For this review, take the finished solid that the model builds, in its own axes (mm). Give positions to 0.01 mm unless a question says otherwise; leave off trailing zeros. Write each loop counter-clockwise with the first axis right and the second up, starting at its lowest first coordinate (ties: lowest second). Pieces come first, ordered by that corner, then holes. Notation, with made-up numbers: (0, 28) -> (35, 28) arc R13 ccw to (35, 42) -> close; hole circle Ø2 at (-21.5, 23). An arc over 180 degrees is marked (long way). Answer as CSV lines item,"result".
Autodesk Inventor part; units mm, degrees
ref_plane "YZ Plane" through (0, 0, 0) normal (1, 0, 0) x (0, 1, 0)
ref_plane "XZ Plane" through (0, 0, 0) normal (0, 1, 0) x (-1, 0, 0)
ref_plane "XY Plane" through (0, 0, 0) normal (0, 0, 1) x (1, 0, 0)
sketch "Sketch1" plane through (0, 0, 0) normal (0, 1, 0) x (-1, 0, 0)
  line L0 (0, 0) -> (1000, 0)
  line L1 (1000, 0) -> (1000, 1500)
  line L2 (1000, 1500) -> (0, 1500)
  line L3 (0, 1500) -> (0, 0)
  dimension "d0" = 1000
  dimension "d1" = 1500
extrude "base" add sketch "Sketch1" along normal blind 150
sketch "Sketch2" plane through (0, 150, 0) normal (0, 1, 0) x (1, 0, 0)
  circle A0 centre (-290, -609) radius 55
  line L0 (0, 0) -> (-1000, 0)
  line L1 (0, -1500) -> (0, 0)
  dimension "d4" = 110
  dimension "d38" = 609
  dimension "d62" = 290
extrude "air" cut sketch "Sketch2" against normal through all
sketch "Sketch6" plane through (0, 150, 0) normal (0, 1, 0) x (1, 0, 0)
  line L0 (-1000, 0) -> (-1000, -1500)
  circle A0 centre (-880, -1350) radius 55
  line L1 (-1000, -1500) -> (0, -1500)
  dimension "d56" = 110
  dimension "d60" = 150
  dimension "d61" = 120
hole "air2" at (-880, 150, 1350) direction (0, -1, 0) diameter 110 end through all
properties part number "plinth" material "Concrete"
Q1. Add section B-B (x = -880). Write out the cut boundary in (y, z), plus the area to 4 significant figures.
Answer block:
outline,"(0, 0) -> (150, 0) -> (150, 1295) -> (0, 1295) -> close; (0, 1405) -> (150, 1405) -> (150, 1500) -> (0, 1500) -> close"
area,"208,500 mm2"
Q2. Draft analysis for pull direction X (two halves, no side actions). For faces 1 (the flat face through (0, 74, 760)), 2 (the flat face through (-1000, 74, 740)), 3 (the flat face through (-507, 74, 1500)), 4 (the cylindrical face through (-264.621, 76.05, 657.794)), state which applies: released by +X, released by -X, zero draft, split by the parting line, or undercut.
Answer block:
face 1,"released by +X"
face 2,"released by -X"
face 3,"zero draft"
face 4,"undercut"
Q3. To check wall thickness, follow probe 1 along Z at (x, y) = (-880, 100.5); probe 2 along Z at (x, y) = (-290, 68); probe 3 along X at (y, z) = (98, 1350). State the ranges of each line that lie inside material, in increasing order. Write a range as [from, to].
Answer block:
probe 1,"z = [0, 1295], [1405, 1500]"
probe 2,"z = [0, 554], [664, 1500]"
probe 3,"x = [-1000, -935], [-825, 0]"
Q4. Add section A-A (z = 1350). Write out the cut boundary in (x, y), plus the area to 4 significant figures.
Answer block:
outline,"(-1000, 0) -> (-935, 0) -> (-935, 150) -> (-1000, 150) -> close; (-825, 0) -> (0, 0) -> (0, 150) -> (-825, 150) -> close"
area,"133,500 mm2"
